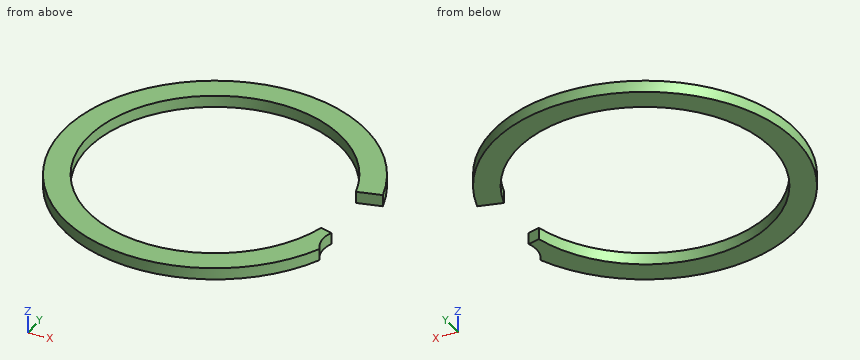
from build123d import *

# Parameters (mm, degrees)
BOSS_EXTRUDE1_DEPTH = 1.15


with BuildPart() as part:
    # Sketch1 → Boss-Extrude1 (new body)
    with BuildSketch(Plane(origin=(0, 0, 0), x_dir=(-1, 0, 0), z_dir=(0, 0, -1))):
        with BuildLine():
            Line((-14.334339262, 3.840874629), (-12.035435796, 3.224885302))
            ThreePointArc((-12.035435796, 3.224885302), (12.46, 0), (-12.035435796, -3.224885302))
            Line((-12.035435796, -3.224885302), (-13.184887529, -3.532879966))
            ThreePointArc((-13.184887529, -3.532879966), (-12.98832562, -4.918513333), (-13.467338447, -6.233489806))
            ThreePointArc((-13.467338447, -6.233489806), (14.785348341, 1.272428564), (-14.334339262, 3.840874629))
        make_face()
    extrude(amount=-BOSS_EXTRUDE1_DEPTH)


solid = part.part
Read the model definition and answer for the solid it produces. Units are mm, in the model's axes. Give positions to 0.01 mm unless a question says otherwise; leave off trailing zeros. Write each loop counter-clockwise with the first axis right and the second up, starting at its lowest first coordinate (ties: lowest second). Pieces come first, ordered by that corner, then holes. Notation, with made-up numbers: (-25.75, 13) - (12.25, 13) arc R26 ccw to (12.25, 45) - close; hole circle Ø2 at (64.25, 76.5). An arc over 180 degrees is marked (long way). Answer in a Markdown table with one row per item. Add a question column.
Item 1: A flat-ended cylindrical pin translates along its axis: P1, Ø8, axis at x = 2.5, y = -7, coming from the -Z side. Find the tip coordinate at first contact, or state that the pin passes through.
Item 2: Section A-A, the plane x = 0 is taken. Write down the section's boundary in (y, z).
Item 3: Section B-B, the plane y = 5.25 is taken. Write down the section's boundary in (x, z), and give its area (3 significant figures).
Item 4: Section C-C, the plane y = 0 is taken. Write down the section's boundary in (x, z), and give its area (3 significant figures).
Item 5: Find the intervals of material crossed by L1, parallel to Y at x = 0, z = 0.9; L2, parallel to X at y = 0, z = 0.4; L3, parallel to X at y = -11.25, z = 0.5, in increasing order.
Recorded:
| question | item | result |
|---|---|---|
| 1 | P1 | passes through |
| 2 | outline | (-14.84, 0) - (-12.46, 0) - (-12.46, 1.15) - (-14.84, 1.15) - close; (12.46, 0) - (14.84, 0) - (14.84, 1.15) - (12.46, 1.15) - close |
| 3 | outline | (-13.88, 0) - (-11.3, 0) - (-11.3, 1.15) - (-13.88, 1.15) - close; (11.3, 0) - (13.88, 0) - (13.88, 1.15) - (11.3, 1.15) - close |
| 3 | area | 5.93 mm2 |
| 4 | outline | (-14.84, 0) - (-12.46, 0) - (-12.46, 1.15) - (-14.84, 1.15) - close |
| 4 | area | 2.74 mm2 |
| 5 | L1 | y = -14.84 to -12.46, 12.46 to 14.84 |
| 5 | L2 | x = -14.84 to -12.46 |
| 5 | L3 | x = -9.68 to -5.36, 5.36 to 9.68 |
